from build123d import *

# Parameters (mm, degrees)
F1_DEPTH = 63.5
F2_DEPTH = 25.4
F3_DEPTH = 15.875
F5_R     = 6.35


with BuildPart() as f1:
    # F0 (on Front) → F1 (new body, symmetric)
    with BuildSketch(Plane.XZ):
        Polygon((30.7617224753, 14.2875), (-44.45, 14.2875), (-44.45, -14.2875), (44.45, -14.2875), (44.45, 14.2875), align=None)
    extrude(amount=F1_DEPTH, both=True)

    # F0 (on Front) → F2 (join, symmetric)
    with BuildSketch(Plane.XZ):
        with BuildLine():
            Line((30.7617224753, 52.3875), (30.7617224753, 14.2875))
            Line((30.7617224753, 14.2875), (44.45, 14.2875))
            Line((44.45, 14.2875), (44.45, 52.3875))
            ThreePointArc((44.45, 52.3875), (49.0996798487, 63.6128201513), (60.325, 68.2625))
            Line((60.325, 68.2625), (75.7897496223, 68.2625))
            Line((75.7897496223, 68.2625), (75.7897496223, 81.9507775247))
            Line((75.7897496223, 81.9507775247), (60.325, 81.9507775247))
            add(Edge.make_bspline(
                [(54.9267858452, 81.4537460931), (56.7210795093, 81.6729876967), (58.5208597277, 81.8394540981), (60.325, 81.9507775247)],
                knots=[119.3724573368, 119.3724573368, 119.3724573368, 119.3724573368, 124.7241746831, 124.7241746831, 124.7241746831, 124.7241746831], degree=3))
            ThreePointArc((54.9267858452, 81.4537460931), (37.5920252585, 71.2872152731), (30.7617224753, 52.3875))
        make_face()
        Polygon((101.1993896154, 81.9507775247), (75.7897496223, 81.9507775247), (75.7897496223, 68.2625), (101.1937051574, 68.2625), align=None)
    extrude(amount=F2_DEPTH, both=True)

    # F0 (on Front) → F3 (join, symmetric)
    with BuildSketch(Plane.XZ):
        with BuildLine():
            add(Edge.make_bspline(
                [(-44.45, 14.2875), (-22.3885229669, 45.4157741444), (14.904260364, 76.5634637243), (54.9267858452, 81.4537460931)],
                knots=[0, 0, 0, 0, 119.3724573368, 119.3724573368, 119.3724573368, 119.3724573368], degree=3))
            Line((-44.45, 14.2875), (30.7617224753, 14.2875))
            Line((30.7617224753, 14.2875), (30.7617224753, 52.3875))
            ThreePointArc((30.7617224753, 52.3875), (37.5920252585, 71.2872152731), (54.9267858452, 81.4537460931))
        make_face()
    extrude(amount=F3_DEPTH, both=True)

    # F0 (on Front) → F4 (revolve)
    with BuildSketch(Plane.XZ):
        Polygon((101.2016162276, 87.3125), (101.1993896154, 81.9507775247), (101.1937051574, 68.2625), (101.1897496223, 58.7375), (126.5897496223, 58.7375), (126.5897496223, 87.3125), align=None)
    revolve(axis=Axis((101.195682925, 0, 73.025), (0.0004152792, 0, 0.9999999138)))

    # F5
    f5_edges = [f1.edges().sort_by_distance(p)[0] for p in [
        (-44.45, 63.5, 0),
        (-44.45, -63.5, 0),
        (44.45, 63.5, 0),
        (44.45, -63.5, 0),
    ]]
    fillet(f5_edges, radius=F5_R)


solid = f1.part
Geometry check sheet. Reference: the model listing, model coordinates, mm. A direction names the side the tool comes from. Coordinates: 2 decimals unless noted, no trailing zeros. Order: outer loops, then holes, each group sorted by start corner. A loop starts at its lowest first (then second) coordinate and runs counter-clockwise, first axis right, second up. Notation, with made-up numbers: (-5, -3.5) -> (53, -3.5) arc R27 ccw to (53, 24.5) -> close; hole circle Ø7 at (69.25, -6). An arc over 180 degrees is marked (long way). Use a Markdown table: item, result. Add a question column.
1. Cross-section at B-B (y = 42). Enter the section's corners in (x, z).
2. Material ranges on L1, parallel to X at y = -6, z = -7; L2, parallel to Z at x = 42.5, y = -49.5; L3, parallel to Z at x = 84, y = 24.5, recorded low to high.
3. Cross-section at A-A (z = -4). Enter the section's corners in (x, y).
4. Set-up check for faces 5 (the face through (30.762, -21, 34)), 6 (the face through (30.762, 21, 34)): record each of +Z, -Z, +X, -X, +Y, -Y from which the full face is reachable in a straight line by a thin tool's end or side.
5. Mould release check, pull along X, two halves, no side actions. Record for faces 1 (the face through (44.45, -1, 11)), 2 (the face through (1, -40, 14.288)), 3 (the face through (-44.45, -1, 0)), 4 (the face through (48.98, -0.36, 63.49)): pulls with the +X half, pulls with the -X half, needs draft (parallel to the pull), parting line crosses it, or undercut.
6. Go/stop test with flat-tipped pins: pin 1 Ø20 at (x, z) = (2.5, 57.5) entering from -Y (3 decimals); pin 2 Ø5 at (y, z) = (-19, 26) entering from -X; pin 3 Ø1.5 at (x, y) = (18.5, 13) entering from +Z; pin 4 Ø1 at (x, z) = (-12.5, 51.5) entering from +Y. Record where each tip stops, or that it passes through.
Filled sheet:
| question | item | result |
|---|---|---|
| 1 | outline | (-44.45, -14.29) -> (44.45, -14.29) -> (44.45, 14.29) -> (-44.45, 14.29) -> close |
| 2 | L1 | -44.45 to 44.45 |
| 2 | L2 | -14.29 to 14.29 |
| 2 | L3 | 68.26 to 81.95 |
| 3 | outline | (-44.45, -57.15) arc R6.35 ccw to (-38.1, -63.5) -> (38.1, -63.5) arc R6.35 ccw to (44.45, -57.15) -> (44.45, 57.15) arc R6.35 ccw to (38.1, 63.5) -> (-38.1, 63.5) arc R6.35 ccw to (-44.45, 57.15) -> close |
| 4 | face 5 | +Z, -X, -Y |
| 4 | face 6 | +Z, -X, +Y |
| 5 | face 1 | pulls with the +X half |
| 5 | face 2 | needs draft |
| 5 | face 3 | pulls with the -X half |
| 5 | face 4 | undercut |
| 6 | pin 1 | y = -15.875 |
| 6 | pin 2 | x = 30.76 |
| 6 | pin 3 | z = 70.31 |
| 6 | pin 4 | through |
